CAD build for the part. Positions are in the model's coordinates, mm. A direction names the side the tool comes from. Give positions to 0.01 mm unless a question says otherwise; leave off trailing zeros. Write each loop counter-clockwise with the first axis right and the second up, starting at its lowest first coordinate (ties: lowest second). Pieces come first, ordered by that corner, then holes. Notation, with made-up numbers: (-20, 64) -> (-6, 64) arc R20 ccw to (-6, 85) -> close; hole circle Ø4 at (55.25, 30). An arc over 180 degrees is marked (long way). Answer as a JSON object with one key per item and string values.
```python
from build123d import *

# Parameters (mm, degrees)
SKETCH1_W                        = 17.78
SKETCH1_H                        = 25.4
EXTRUDE1_DEPTH                   = 10.16
F_3_8_0_375_DIAMETER_HOLE1_D     = 9.525
F_3_8_0_375_DIAMETER_HOLE1_DEPTH = 12.7
F_3_8_0_375_DIAMETER_HOLE1_TIP   = 2.861598698
SKETCH11_OUTSIDE_W               = 26.306
SKETCH11_OUTSIDE_H               = 33.926
SKETCH11_OUTSIDE_R               = 6.35
EXTRUDE3_DEPTH                   = 5.08
F_39_0_0995_DIAMETER_HOLE1_D     = 2.5273
SKETCH14_W                       = 6.858
SKETCH14_H                       = 6.858
EXTRUDE4_DEPTH                   = 6.08


with BuildPart() as part:
    # Sketch1 → Extrude1 (new body)
    with BuildSketch(Plane.XY):
        Rectangle(SKETCH1_W, SKETCH1_H)
    extrude(amount=EXTRUDE1_DEPTH)

    # 3/8 (0.375) Diameter Hole1
    with Locations(Plane(origin=(-2.54, 0, 10.16), x_dir=(1, 0, 0), z_dir=(0, 0, 1))):
        with Locations((0, 0)):
            Hole(F_3_8_0_375_DIAMETER_HOLE1_D / 2, depth=F_3_8_0_375_DIAMETER_HOLE1_DEPTH)
            with Locations((0, 0, -(F_3_8_0_375_DIAMETER_HOLE1_DEPTH + F_3_8_0_375_DIAMETER_HOLE1_TIP / 2))):  # 118° drill point
                Cone(0, F_3_8_0_375_DIAMETER_HOLE1_D / 2, F_3_8_0_375_DIAMETER_HOLE1_TIP, mode=Mode.SUBTRACT)

    # Sketch11 outside → Extrude3 (cut)
    with BuildSketch(Plane.XY.offset(10.16)):
        Rectangle(SKETCH11_OUTSIDE_W, SKETCH11_OUTSIDE_H)
        with Locations((-2.54, 0)):
            Circle(SKETCH11_OUTSIDE_R, mode=Mode.SUBTRACT)
    extrude(amount=-EXTRUDE3_DEPTH, mode=Mode.SUBTRACT)

    # #39 (0.0995) Diameter Hole1 (through all)
    with Locations(Plane(origin=(6.858, 0, 10.16), x_dir=(1, 0, 0), z_dir=(0, 0, 1))):
        with Locations((0, 0), (-9.398, -9.398), (-9.398, 9.398)):
            Hole(F_39_0_0995_DIAMETER_HOLE1_D / 2)

    # Sketch14 → Extrude4 (cut, through all)
    with BuildSketch(Plane.XY.offset(5.08)):
        with Locations((5.461, 9.271)):
            Rectangle(SKETCH14_W, SKETCH14_H)
        with Locations((5.461, -9.271)):
            Rectangle(SKETCH14_W, SKETCH14_H)
    extrude(amount=-EXTRUDE4_DEPTH, mode=Mode.SUBTRACT)


solid = part.part
```
1) Slice it at D-D (y = -1). List the corners of the cut face in (x, z).
Model answer:
{"outline": "(-8.89, 0) -> (-7.2, 0) -> (-7.2, 10.16) -> (-8.81, 10.16) -> (-8.81, 5.08) -> (-8.89, 5.08) -> close; (2.12, 0) -> (6.09, 0) -> (6.09, 5.08) -> (3.73, 5.08) -> (3.73, 10.16) -> (2.12, 10.16) -> close; (7.63, 0) -> (8.89, 0) -> (8.89, 5.08) -> (7.63, 5.08) -> close"}
2) Slice it at A-A (x = -2.54). List the corners of the cut face in (y, z), then the cut area to 3 significant figures.
Model answer:
{"outline": "(-12.7, 0) -> (-10.66, 0) -> (-10.66, 5.08) -> (-12.7, 5.08) -> close; (-8.13, 0) -> (-4.76, 0) -> (-4.76, 10.16) -> (-6.35, 10.16) -> (-6.35, 5.08) -> (-8.13, 5.08) -> close; (4.76, 0) -> (8.13, 0) -> (8.13, 5.08) -> (6.35, 5.08) -> (6.35, 10.16) -> (4.76, 10.16) -> close; (10.66, 0) -> (12.7, 0) -> (12.7, 5.08) -> (10.66, 5.08) -> close", "area": "71.1 mm2"}
3) 3-axis set-ups, long thin cutter, end or side, ignore diameter. For faces 4 (the flat face through (2.032, 9, 3)), 5 (the flat face through (5, -5.842, 3)), 6 (the flat face through (-4, -12.7, 3)): which of +Z, -Z, +X, -X, +Y, -Y reach the whole face in a straight line?
Model answer:
{"face 4": "+Z, -Z, +X, +Y", "face 5": "+Z, -Z, +X, -Y", "face 6": "+Z, -Z, +X, -X, -Y"}
4) Wall check: probe 1 along Y at (x, z) = (-2.54, 3.55); probe 2 along Z at (x, y) = (-6, 10.25); probe 3 along Y at (x, z) = (1, 0.75). Give the ranges that are in metal, low to high.
Model answer:
{"probe 1": "y = -12.7 to -10.66, -8.13 to -4.76, 4.76 to 8.13, 10.66 to 12.7", "probe 2": "z = 0 to 5.08", "probe 3": "y = -12.7 to -3.19, 3.19 to 12.7"}
5) Pin check, flat tips, straight feed: pin 1 (2.5 mm diameter, centred on y = -10.5, z = 3, fed in from +X); pin 2 (5.5 mm diameter, centred on x = -1, y = -1, fed in from +Z); pin 3 (5.5 mm diameter, centred on x = 5.5, z = 3.5, fed in from +Y); pin 4 (3.5 mm diameter, centred on x = -2.54, y = 9.398, fed in from +Z). Stop position of each tip, or through.
Model answer:
{"pin 1": "stops at x = 2.03", "pin 2": "passes through", "pin 3": "stops at y = 5.84", "pin 4": "stops at z = 5.08"}
6) Mould opens along X. For faces 1 (the cylindrical face through (-3.92, -6.2, 7.66)), 2 (the flat face through (2, 3, 0)), 3 (the cylindrical face through (1.24, -2.9, 5.01)) say: released by +X, released by -X, zero draft, split by the parting line, or undercut.
Model answer:
{"face 1": "split by the parting line", "face 2": "zero draft", "face 3": "undercut"}
7) Slice it at B-B (x = -5). List the corners of the cut face in (y, z).
Model answer:
{"outline": "(-12.7, 0) -> (-4.08, 0) -> (-4.08, 10.16) -> (-5.85, 10.16) -> (-5.85, 5.08) -> (-12.7, 5.08) -> close; (4.08, 0) -> (12.7, 0) -> (12.7, 5.08) -> (5.85, 5.08) -> (5.85, 10.16) -> (4.08, 10.16) -> close"}
